```python
from build123d import *

# Parameters (mm, degrees)
F1_DEPTH      = 49
F2_W          = 7.5
F2_H          = 9.53
F3_DEPTH      = 2.4
F4_W          = 1.362546
F4_H          = 4.923334
F5_DEPTH      = 9
F5_DEPTH_BACK = 58.4


with BuildPart() as f1:
    # F0 (on Front) → F1 (new body)
    with BuildSketch(Plane.XZ):
        Polygon((-15.2, 0), (0, 0), (0, 2.41), (0, 10.307252), (-1.6, 14.3), (-13.6, 14.3), (-15.2, 10.307252), (-15.2, 2.41), align=None)
    extrude(amount=F1_DEPTH)

    # F2 (on face) → F3 (join)
    with BuildSketch(Plane(origin=(0, 0, 0), x_dir=(1, 0, 0), z_dir=(0, 0, -1))):
        with Locations((-18.95, 4.765)):
            Rectangle(F2_W, F2_H)
        with Locations((3.75, 44.235)):
            Rectangle(F2_W, F2_H)
    extrude(amount=-F3_DEPTH)

    # F4 (on face) → F5 (join, two sides)
    with BuildSketch(Plane(origin=(0, 0, 0), x_dir=(-1, 0, 0), z_dir=(0, 1, 0))) as f5_sk:
        with Locations((7.6, 7.15)):
            Rectangle(F4_W, F4_H)
    extrude(amount=F5_DEPTH)
    extrude(f5_sk.sketch, amount=-F5_DEPTH_BACK)


solid = f1.part
```
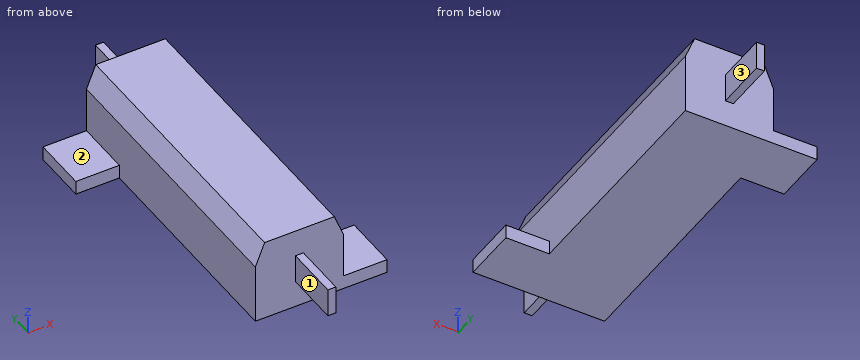
Check sheet for the modelled part. Datum: model origin and axes. Units: mm. Face numbers are marked on the shaded views. A direction names the side the tool comes from. Give positions to 0.01 mm unless a question says otherwise; leave off trailing zeros. Write each loop counter-clockwise with the first axis right and the second up, starting at its lowest first coordinate (ties: lowest second). Pieces come first, ordered by that corner, then holes.
Item 1: Cross-section at C-C (x = -3). Enter the section's corners in (y, z), and give its area (3 significant figures).
Item 2: Access from +Z, -Z, +X, -X, +Y, -Y to the whole of each face (thin tool, end or side, straight path). Record for the marked faces 1, 2 and 3.
Item 3: Gauge pin test, flat ends, axial feed: pin 1 (6 mm diameter, centred on x = -19, y = -4.5, fed in from +Z); pin 2 (0.7 mm diameter, centred on x = -8, y = -54.5, fed in from -Z); pin 3 (0.7 mm diameter, centred on x = -7.5, y = -55, fed in from +Z). Record the tip position at first contact, or that the pin passes through.
Item 4: Scan lines: L1, parallel to Y at x = -4.5, z = 2; L2, parallel to X at y = -1.5, z = 1; L3, parallel to X at y = -3, z = 2.5. Record each from-to range of solid material in increasing order.
Item 5: Cross-section at B-B (y = -30.5). Enter the section's corners in (x, z), and give its area (3 significant figures).
Item 6: Cross-section at A-A (z = 8.5). Enter the section's corners in (x, y).
Item 7: Cross-section at D-D (y = -8.5). Enter the section's corners in (x, z), and give its area (3 significant figures).
Report:
1. outline: (-49, 0) - (0, 0) - (0, 14.3) - (-49, 14.3) - close
1. area: 701 mm2
2. face 1: +Z, -Z, -X, -Y
2. face 2: +Z, -X, +Y, -Y
2. face 3: +Z, -Z, +X, +Y
3. pin 1: stops at z = 2.4
3. pin 2: stops at z = 4.69
3. pin 3: stops at z = 9.61
4. L1: y = -49 to 0
4. L2: x = -22.7 to 0
4. L3: x = -15.2 to 0
5. outline: (-15.2, 0) - (0, 0) - (0, 10.31) - (-1.6, 14.3) - (-13.6, 14.3) - (-15.2, 10.31) - close
5. area: 211 mm2
6. outline: (-15.2, -49) - (-8.28, -49) - (-8.28, -58.4) - (-6.92, -58.4) - (-6.92, -49) - (0, -49) - (0, 0) - (-6.92, 0) - (-6.92, 9) - (-8.28, 9) - (-8.28, 0) - (-15.2, 0) - close
7. outline: (-22.7, 0) - (0, 0) - (0, 10.31) - (-1.6, 14.3) - (-13.6, 14.3) - (-15.2, 10.31) - (-15.2, 2.4) - (-22.7, 2.4) - close
7. area: 229 mm2
